The drawing under review shows one solid part. Ordinate dimensions are in mm from its lowest x, y, z. Give positions to 0.01 mm unless a question says otherwise; leave off trailing zeros. Write each loop counter-clockwise with the first axis right and the second up, starting at its lowest first coordinate (ties: lowest second). Pieces come first, ordered by that corner, then holes.
Q1. We need section B-B (z = 3.5). Write out the cut boundary in (x, y), then the cut area to 3 significant figures.
Q2. For line 1 (Y direction, x = 74, z = 3.2); line 2 (X direction, y = 72.5, z = 2.2); line 3 (Y direction, x = 66, z = 1.95), list the stretches that pass through material, from the lowest coordinate up.
Q3. We need section A-A (y = 74). Write out the cut boundary in (x, z), then the cut area to 3 significant figures.
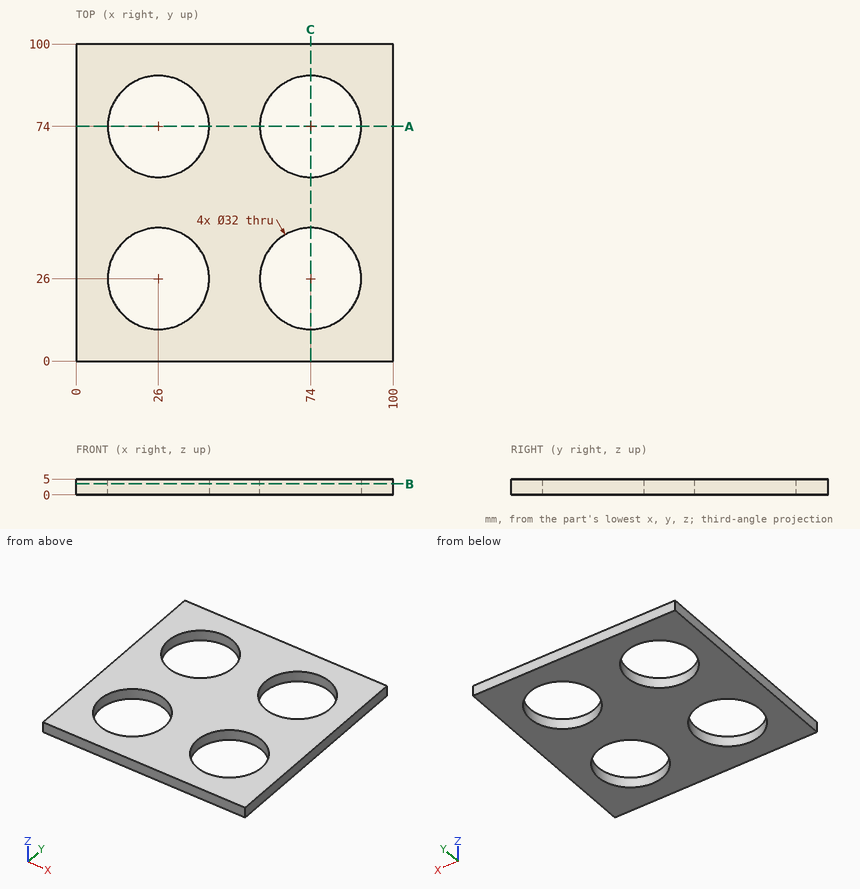
Computed:
1. outline: (0, 0) - (100, 0) - (100, 100) - (0, 100) - close; hole circle Ø32 at (26, 26); hole circle Ø32 at (26, 74); hole circle Ø32 at (74, 26); hole circle Ø32 at (74, 74)
1. area: 6,780 mm2
2. line 1: y = 0 to 10, 42 to 58, 90 to 100
2. line 2: x = 0 to 10.07, 41.93 to 58.07, 89.93 to 100
2. line 3: y = 0 to 12.14, 39.86 to 60.14, 87.86 to 100
3. outline: (0, 0) - (10, 0) - (10, 5) - (0, 5) - close; (42, 0) - (58, 0) - (58, 5) - (42, 5) - close; (90, 0) - (100, 0) - (100, 5) - (90, 5) - close
3. area: 180 mm2
